Here's how the part is built. I have some questions about the finished solid (model axes, mm). A direction names the side the tool comes from. Round coordinates to 2 decimals unless told otherwise and drop trailing zeros. Order: outer loops, then holes, each group sorted by start corner. A loop starts at its lowest first (then second) coordinate and runs counter-clockwise, first axis right, second up.
```python
from build123d import *

# Parameters (mm, degrees)
EXTRUDE_1_DEPTH      = 6
SKETCH_5_3_OUTSIDE_W = 103.914
SKETCH_5_3_OUTSIDE_H = 103.914
SKETCH_5_3_OUTSIDE_R = 8.5
CUT_EXTRUDE_1_DEPTH  = 8
CUT_EXTRUDE_1_DRAFT  = -60
CUT_EXTRUDE_START    = -6
SKETCH_5_4_OUTSIDE_W = 103.914
SKETCH_5_4_OUTSIDE_H = 103.914
SKETCH_5_4_OUTSIDE_R = 8.5
CUT_EXTRUDE_2_DEPTH  = 8
CUT_EXTRUDE_2_DRAFT  = 60
CUT_EXTRUDE_START_2  = -8
CUT_EXTRUDE_3_DEPTH  = 8
CHAMFER_1_SIZE       = 1


with BuildPart() as part:
    # 草图4 → 旋转1 (revolve)
    with BuildSketch(Plane(origin=(0, 0, 0), x_dir=(0, 0, -1), z_dir=(1, 0, 0)), mode=Mode.PRIVATE) as revolve_1_sk:
        Polygon((206.9, 6), (206.9, 15), (216.9, 15), (216.9, 0), (0, 0), (0, 5), (22, 5), (22, 6), align=None)
    revolve(revolve_1_sk.sketch.rotate(Axis((0, 0, -216.9), (0, 0, 1)), 90), axis=Axis((0, 0, -216.9), (0, 0, 1)))

    # 草图6 → 切除-拉伸3 (cut)
    with BuildSketch(Plane.XY.offset(-22).offset(CUT_EXTRUDE_START_2)):
        with BuildLine():
            ThreePointArc((3.31662479, 5), (0, 6), (-3.31662479, 5))
            Line((-3.31662479, 5), (3.31662479, 5))
        make_face()
        with BuildLine():
            ThreePointArc((6, 0), (5.744562647, 1.732050808), (5, 3.31662479))
            Line((5, 3.31662479), (5, -3.31662479))
            ThreePointArc((5, -3.31662479), (5.744562647, -1.732050808), (6, 0))
        make_face()
        with BuildLine():
            Line((3.31662479, -5), (-3.31662479, -5))
            ThreePointArc((-3.31662479, -5), (0, -6), (3.31662479, -5))
        make_face()
        with BuildLine():
            Line((-5, -3.31662479), (-5, 3.31662479))
            ThreePointArc((-5, 3.31662479), (-6, 0), (-5, -3.31662479))
        make_face()
    extrude(amount=CUT_EXTRUDE_3_DEPTH, mode=Mode.SUBTRACT)

    # 倒角1
    chamfer_1_edges = [part.edges().sort_by_distance(p)[0] for p in [
        (5, 0, 0),
    ]]
    chamfer(chamfer_1_edges, length=CHAMFER_1_SIZE)


with BuildPart() as body_2:
    # 草图5 → 凸台-拉伸1 (new body)
    with BuildSketch(Plane.XY.offset(-11)):
        Polygon((0, 9.814954576), (-8.5, 4.907477288), (-8.5, -4.907477288), (0, -9.814954576), (8.5, -4.907477288), (8.5, 4.907477288), align=None)
    extrude(amount=-EXTRUDE_1_DEPTH)


with BuildPart() as cut_extrude_1_tool:
    # 草图5<3> outside → 切除-拉伸1 (with draft: the straight prism first)
    with BuildSketch(Plane.XY.offset(-11)):
        Rectangle(SKETCH_5_3_OUTSIDE_W, SKETCH_5_3_OUTSIDE_H)
        Circle(SKETCH_5_3_OUTSIDE_R, mode=Mode.SUBTRACT)
    extrude(amount=-CUT_EXTRUDE_1_DEPTH)
    # 切除-拉伸1: the draft: its side faces are tilted about the plane it starts from
    cut_extrude_1_sides = [cut_extrude_1_tool.faces().sort_by_distance(p)[0] for p in [
        (0, -51.957, -15),
        (51.957, 0, -15),
        (0, 51.957, -15),
        (-51.957, 0, -15),
        (-8.5, 0, -15),
    ]]
    draft(cut_extrude_1_sides, Plane.XY.offset(-11), CUT_EXTRUDE_1_DRAFT)


with BuildPart() as body_2_1:
    add(body_2.part)

    # 切除-拉伸1: cut by cut_extrude_1_tool
    add(cut_extrude_1_tool.part, mode=Mode.SUBTRACT)


with BuildPart() as cut_extrude_2_tool:
    # 草图5<4> outside → 切除-拉伸2 (with draft: the straight prism first)
    with BuildSketch(Plane.XY.offset(-11).offset(CUT_EXTRUDE_START)):
        Rectangle(SKETCH_5_4_OUTSIDE_W, SKETCH_5_4_OUTSIDE_H)
        Circle(SKETCH_5_4_OUTSIDE_R, mode=Mode.SUBTRACT)
    extrude(amount=CUT_EXTRUDE_2_DEPTH)
    # 切除-拉伸2: the draft: its side faces are tilted about the plane it starts from
    cut_extrude_2_sides = [cut_extrude_2_tool.faces().sort_by_distance(p)[0] for p in [
        (0, -51.957, -13),
        (51.957, 0, -13),
        (0, 51.957, -13),
        (-51.957, 0, -13),
        (-8.5, 0, -13),
    ]]
    draft(cut_extrude_2_sides, Plane.XY.offset(-11).offset(CUT_EXTRUDE_START), CUT_EXTRUDE_2_DRAFT)


with BuildPart() as body_2_2:
    add(body_2_1.part)

    # 切除-拉伸2: cut by cut_extrude_2_tool
    add(cut_extrude_2_tool.part, mode=Mode.SUBTRACT)

    # Combine 1: union part
    add(part.part)


solid = body_2_2.part
```
1. I'm going to push flat-ended pins straight in: P1, Ø0.5, axis at x = 5.5, y = 1, coming from the +Z side; P2, Ø3.5, axis at y = -1, z = -26.5, coming from the -X side; P3, Ø6, axis at y = -8.5, z = -116.5, coming from the -X side; P4, Ø6, axis at y = -10.5, z = -155, coming from the -X side. Where does each tip first touch, or does it pass through?
Evaluation:
P1: stops at z = -11
P2: stops at x = -5
P3: stops at x = -2.4
P4: passes through
2. On a 3-axis mill with a long thin cutter (end or side, diameter ignored), from which of +Z, -Z, +X, -X, +Y, -Y can I reach the whole of each face in a straight line? I mean faces 4 (the flat face through (0, 5, -26)), 5 (the flat face through (-4, 4, -22)), 6 (the flat face through (-5, 0, -26)), 7 (the conical face through (7.64, 4.39, -16.82)), 8 (the conical face through (7.62, -4.43, -16.82)). Say none if no direction works.
Evaluation:
face 4: +X, -X, +Y
face 5: -X, +Y
face 6: -X, +Y, -Y
face 7: +X, +Y
face 8: +X, -Y
3. I need wall thicknesses on probe 1 along X at (y, z) = (0, -71); probe 2 along Z at (x, y) = (11.25, 3.5); probe 3 along Y at (x, z) = (5, -146). Which ranges of each line are inside material? Lowest first, please.
Evaluation:
probe 1: x = -6 to 6
probe 2: z = -216.9 to -206.9
probe 3: y = -3.32 to 3.32
4. If we mould it in two halves opening along Z, with no side actions, what happens to faces 1 (the flat face through (0, 0, -216.9)), 2 (the flat face through (0, -5, -26)), 3 (the conical face through (-7.62, 4.43, -11.18))? For each: released by +Z, released by -Z, zero draft, split by the parting line, or undercut.
Evaluation:
face 1: released by -Z
face 2: undercut
face 3: released by +Z
5. If we section it at A-A, the plane z = -32.5: Write out the boundary of the cut face in (x, y), and give its area (3 significant figures).
Evaluation:
outline: circle Ø12 at (0, 0)
area: 113 mm2
6. If we section it at B-B, the plane x = 12.5: Write out the boundary of the cut face in (y, z).
Evaluation:
outline: (-8.29, -216.9) - (8.29, -216.9) - (8.29, -206.9) - (-8.29, -206.9) - close
